Autodesk Inventor part; units mm, degrees
ref_plane "YZ Plane" through (0, 0, 0) normal (1, 0, 0) x (0, 1, 0)
ref_plane "XZ Plane" through (0, 0, 0) normal (0, 1, 0) x (-1, 0, 0)
ref_plane "XY Plane" through (0, 0, 0) normal (0, 0, 1) x (1, 0, 0)
sketch "Skizze1" plane through (0, 0, 0) normal (1, 0, 0) x (0, 1, 0)
  circle A0 centre (0, 0) radius 10
  line L0 (-9.8543, 1.7009) -> (-1.1444, 9.9343)
  line L1 (9.8543, -1.7009) -> (1.1444, -9.9343)
  dimension "d0" = 20
extrude "Extrusion1" add sketch "Skizze1" along normal blind 30 contours A0 L1 L0
sketch "Skizze2" plane through (30, 0, 0) normal (1, 0, 0) x (0, -0.687, 0.7267)
  circle A0 centre (0, 0) radius 10
  circle A1 centre (0, 0) radius 1
  dimension "d3" = 2
extrude "Extrusion2" add sketch "Skizze2" along normal blind 7 contours A1
properties part number "motor"
Source: CAD feature listing. Evaluate the final solid. Frame: model axes, mm. A direction names the side the tool comes from. Give positions to 0.01 mm unless a question says otherwise; leave off trailing zeros. Write each loop counter-clockwise with the first axis right and the second up, starting at its lowest first coordinate (ties: lowest second). Pieces come first, ordered by that corner, then holes. Notation, with made-up numbers: M 13,-39 L 55,-39 A21 cw 55,-29 Z; hole C -6.5,-21.75 d9. An arc over 180 degrees is marked long. Return JSON: item names as keys, results as strings. Group by question number.
1) Pin query (flat end, axial travel): P1, Ø5, axis at x = 29.5, z = -4.5, coming from the +Y side; P2, Ø2, axis at x = 8.5, z = 7.5, coming from the -Y side; P3, Ø8, axis at y = -4.5, z = -4, coming from the -X side; P4, Ø1, axis at x = 4.5, z = -8, coming from the +Y side. Return the tip coordinate at first contact, or that it passes through.
2) Material intervals for line 1 along X through (y, z) = (-8, 3); line 2 along Z through (x, y) = (19, -2.75); line 3 along Y through (x, z) = (3.5, 7), sorted ascending. Write a range as [from, to].
3) Cut plane D-D, the plane z = 6.5. Output: boundary loops of the cut face in (x, y).
4) Cut plane A-A, the plane y = 0. Output: boundary loops of the cut face in (x, z), plus the area to 3 significant figures.
5) Cut plane C-C, the plane x = 33. Output: boundary loops of the cut face in (y, z), plus the area to 3 significant figures.
6) Set-up query: faces 1 (the face through (14.79, -5.56, 5.76)), 2 (the face through (33, -1, 0)). Return all of +Z, -Z, +X, -X, +Y, -Y with unobstructed straight access to the full face (end or side cutting, diameter ignored); none if empty.
Recorded:
{
 "1": {"P1": "stops at y = 9.54", "P2": "stops at y = -4.78", "P3": "stops at x = 0", "P4": "stops at y = 3.72"},
 "2": {"line 1": "x = [0, 30]", "line 2": "z = [-9.61, 8.42]", "line 3": "y = [-4.25, 7.14]"},
 "3": {"outline": "M 0,-4.78 L 30,-4.78 L 30,7.6 L 0,7.6 Z"},
 "4": {"outline": "M 0,-10 L 30,-10 L 30,-1 L 37,-1 L 37,1 L 30,1 L 30,10 L 0,10 Z", "area": "614 mm²"},
 "5": {"outline": "C 0,0 d2", "area": "3.14 mm²"},
 "6": {"face 1": "+Z, +X, -X, -Y", "face 2": "+X"}
}
